Verification items for the finished model (mm, model axes). A direction names the side the tool comes from. Round coordinates to 2 decimals unless told otherwise and drop trailing zeros. Write each loop counter-clockwise with the first axis right and the second up, starting at its lowest first coordinate (ties: lowest second). Pieces come first, ordered by that corner, then holes. Notation, with made-up numbers: M -22.75,-1 L -5.75,-1 A32 cw -5.75,34 Z; hole C -19,19.5 d2. An arc over 180 degrees is marked long. Answer in a Markdown table with one row per item. Add a question column.
1. Draft check along Y on faces 1 (the flat face through (-2, -1, 6)), 2 (the cylindrical face through (-2, 0, 3)), 3 (the cylindrical face through (-3.2, -2.4, 3)). Enter one of: pulls with the +Y half, pulls with the -Y half, needs draft (parallel to the pull), parting line crosses it, or undercut.
2. Sectioned sample at B-B on y = 0. Record the cut outline in (x, z), plus the area to 3 significant figures.
3. Sectioned sample at C-C on y = -1.75. Record the cut outline in (x, z), plus the area to 3 significant figures.
4. Material ranges on probe 1 along Y at (x, z) = (-1.5, 2.5); probe 2 along Y at (x, z) = (0, 4.75), recorded low to high.
5. Sectioned sample at D-D on z = 3.5. Record the cut outline in (x, y), plus the area to 3 significant figures.
6. Set-up check for faces 4 (the flat face through (-2, -1, 0)), 5 (the cylindrical face through (2.64, -1.01, 1.89)): record each of +Z, -Z, +X, -X, +Y, -Y from which the full face is reachable in a straight line by a thin tool's end or side.
7. Go/stop test with flat-tipped pins: pin 1 Ø2 at (y, z) = (3, 5) entering from +X; pin 2 Ø3 at (y, z) = (-2, 2.5) entering from +X; pin 3 Ø2.5 at (y, z) = (0, 3) entering from +X. Record where each tip stops, or that it passes through.
8. Sectioned sample at A-A on x = 0. Record the cut outline in (y, z).
```python
from build123d import *

# Parameters (mm, degrees)
SKETCH_1_R           = 4
SKETCH_1_R_2         = 2.025
EXTRUDE_6_DEPTH      = 6
MOVE_FACE_D4_BY      = 0.025
SKETCH_2_R           = 1.5
CUT_EXTRUDE_M3_DEPTH = 9.246211251


with BuildPart() as part:
    # 草图1 → 轴向尺寸_6 (new body)
    with BuildSketch(Plane.XY):
        Circle(SKETCH_1_R)
        Circle(SKETCH_1_R_2, mode=Mode.SUBTRACT)
    extrude(amount=EXTRUDE_6_DEPTH)

    # Move Face D4: a curved face moved outward by 0.025
    add(Solid.thicken(part.faces().sort_by_distance((-2.025, 0, 3))[0], MOVE_FACE_D4_BY))

    # 草图2 → 径向M3螺纹大径包络 (cut, through all)
    with BuildSketch(Plane(origin=(0, 0, 0), x_dir=(0, 0, -1), z_dir=(1, 0, 0))):
        with Locations(Location((-3, 0, 0), (0, 0, 180))):
            Circle(SKETCH_2_R)
    extrude(amount=CUT_EXTRUDE_M3_DEPTH, mode=Mode.SUBTRACT)


solid = part.part
```
Geometry check:
| question | item | result |
|---|---|---|
| 1 | face 1 | needs draft |
| 1 | face 2 | undercut |
| 1 | face 3 | parting line crosses it |
| 2 | outline | M -4,0 L -2,0 L -2,6 L -4,6 Z; M 2,0 L 4,0 L 4,1.5 L 2,1.5 Z; M 2,4.5 L 4,4.5 L 4,6 L 2,6 Z |
| 2 | area | 18.0 mm2 |
| 3 | outline | M -3.6,0 L -0.97,0 L -0.97,6 L -3.6,6 Z; M 0.97,0 L 3.6,0 L 3.6,6 L 0.97,6 Z |
| 3 | area | 31.5 mm2 |
| 4 | probe 1 | y = -3.71 to -1.32, 1.32 to 3.71 |
| 4 | probe 2 | y = -4 to -2, 2 to 4 |
| 5 | outline | M 1.41,-1.41 A2 cw long 1.41,1.41 L 3.74,1.41 A4 ccw long 3.74,-1.41 Z |
| 5 | area | 31.8 mm2 |
| 6 | face 4 | -Z, +X, -X, +Y, -Y |
| 6 | face 5 | +X |
| 7 | pin 1 | stops at x = 3.46 |
| 7 | pin 2 | stops at x = 3.93 |
| 7 | pin 3 | stops at x = -1.56 |
| 8 | outline | M -4,0 L -2,0 L -2,6 L -4,6 Z; M 2,0 L 4,0 L 4,6 L 2,6 Z |
